Geometry: final body of the model. Coordinates: model frame, mm. Face numbers are marked on the shaded views. A direction names the side the tool comes from. Give positions to 0.01 mm unless a question says otherwise; leave off trailing zeros. Loops run counter-clockwise (first coordinate to the right, second up) from the corner with the lowest first, then second, coordinate; pieces in that order, holes last. Notation, with made-up numbers: (-15, 27.25) -> (42, 27.25) arc R28 cw to (42, 64.25) -> close; hole circle Ø9 at (44, 60.5). An arc over 180 degrees is marked (long way). Answer in a Markdown table with one row per item. Add a question column.
1) Access query for the marked faces 1, 2 and 3. Directions: +Z, -Z, +X, -X, +Y, -Y. A direction counts if a zero-diameter tool reaches every point of the face in a straight line with its end or side. Return the directions, or none.
2) Section query D-D (y = -2.75). Return the cut outline in (x, z).
3) Draft query along Z for the marked faces 4, 5, 6 and 7. Return one class per face: +Z half, -Z half, draft (parallel to the pull), parting line (faces both ways), or undercut.
4) First-contact query: P1, Ø1.2, axis at x = 12.5, y = -1, coming from the +Z side; P2, Ø3, axis at x = 12, z = 5.5, coming from the -Y side; P3, Ø1.5, axis at x = -1.5, y = 1.5, coming from the -Z side; P4, Ø3.5, axis at x = 13.5, z = 4.5, coming from the +Y side. Flat tips, straight axial feed; report the tip coordinate or a pass-through.
5) Line query: line 1 (Y direction, x = -3.25, z = 3.25); line 2 (X direction, y = -1.5, z = 4); line 3 (X direction, y = -0.5, z = 6.5). Output: solid intervals per line, ascending. Write a range as from..to.
6) Section query B-B (x = -7.25). Return the cut outline in (y, z), plus the area to 3 significant figures.
7) Section query A-A (z = 3.75). Return the cut outline in (x, y).
8) Section query C-C (x = 15.5). Return the cut outline in (y, z).
```python
from build123d import *

# Parameters (mm, degrees)
SKETCH2_W           = 20
SKETCH2_H           = 9
BOSS_EXTRUDE1_DEPTH = 8
SKETCH3_W           = 4
SKETCH3_H           = 5
CUT_EXTRUDE1_DEPTH  = 10
SKETCH4_W           = 3
SKETCH4_H           = 4
BOSS_EXTRUDE2_DEPTH = 7


with BuildPart() as part:
    # Sketch2 → Boss-Extrude1 (new body)
    with BuildSketch(Plane.XY):
        Rectangle(SKETCH2_W, SKETCH2_H)
    extrude(amount=BOSS_EXTRUDE1_DEPTH)

    # Sketch3 → Cut-Extrude1 (cut)
    with BuildSketch(Plane.ZY.offset(10)):
        with Locations((4, 0)):
            Rectangle(SKETCH3_W, SKETCH3_H)
    extrude(amount=-CUT_EXTRUDE1_DEPTH, mode=Mode.SUBTRACT)

    # Sketch4 → Boss-Extrude2 (add)
    with BuildSketch(Plane(origin=(10, 0, 0), x_dir=(0, 0, -1), z_dir=(1, 0, 0))):
        with Locations((-4, 0)):
            Rectangle(SKETCH4_W, SKETCH4_H)
    extrude(amount=BOSS_EXTRUDE2_DEPTH)


solid = part.part
```
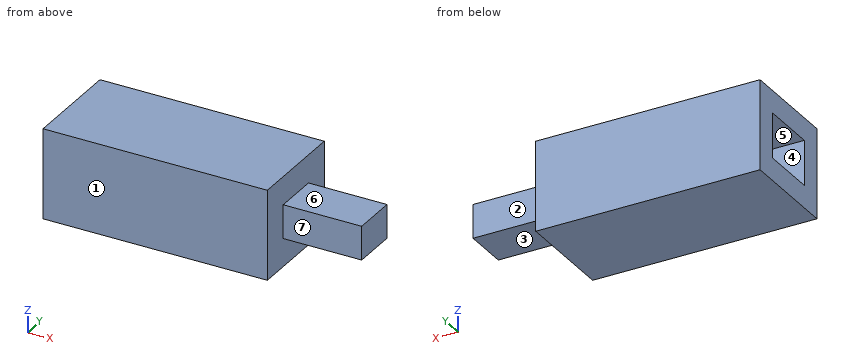
Evaluation:
| question | item | result |
|---|---|---|
| 1 | face 1 | +Z, -Z, +X, -X, -Y |
| 1 | face 2 | +Z, -Z, +X, +Y |
| 1 | face 3 | -Z, +X, +Y, -Y |
| 2 | outline | (-10, 0) -> (10, 0) -> (10, 8) -> (-10, 8) -> close |
| 3 | face 4 | undercut |
| 3 | face 5 | undercut |
| 3 | face 6 | +Z half |
| 3 | face 7 | draft |
| 4 | P1 | z = 5.5 |
| 4 | P2 | y = -2 |
| 4 | P3 | z = 0 |
| 4 | P4 | y = 2 |
| 5 | line 1 | -4.5..-2.5, 2.5..4.5 |
| 5 | line 2 | 0..17 |
| 5 | line 3 | -10..10 |
| 6 | outline | (-4.5, 0) -> (4.5, 0) -> (4.5, 8) -> (-4.5, 8) -> close; hole (-2.5, 2) -> (2.5, 2) -> (2.5, 6) -> (-2.5, 6) -> close |
| 6 | area | 52.0 mm² |
| 7 | outline | (-10, -4.5) -> (10, -4.5) -> (10, -2) -> (17, -2) -> (17, 2) -> (10, 2) -> (10, 4.5) -> (-10, 4.5) -> (-10, 2.5) -> (0, 2.5) -> (0, -2.5) -> (-10, -2.5) -> close |
| 8 | outline | (-2, 2.5) -> (2, 2.5) -> (2, 5.5) -> (-2, 5.5) -> close |
